Can you work these out from the model? Positions are in its coordinate system, mm. Face numbers are marked on the shaded views. Round coordinates to 2 decimals unless told otherwise and drop trailing zeros. Loops run counter-clockwise (first coordinate to the right, second up) from the corner with the lowest first, then second, coordinate; pieces in that order, holes last. Notation, with made-up numbers: M 45,81.5 L 49,81.5 A21 cw 49,87.5 Z; hole C -21.5,82 d10. An arc over 180 degrees is marked long. Use a Markdown table: item, result. Add a question column.
```python
from build123d import *

# Parameters (mm, degrees)
BOSS_EXTRUDE2_DEPTH = 160
SKETCH10_R          = 7.5
CUT_EXTRUDE3_DEPTH  = 37
SKETCH15_W          = 49.972994953
SKETCH15_H          = 20
BOSS_EXTRUDE3_DEPTH = 50
FILLET8_R           = 25
FILLET9_R           = 25
FILLET10_R          = 25
FILLET11_R          = 25
SKETCH20_R          = 12.5
CUT_EXTRUDE16_DEPTH = 120


with BuildPart() as part:
    # Sketch9 → Boss-Extrude2 (new body)
    with BuildSketch(Plane.XY):
        Polygon((-46.127266272, 8.011064826), (33.872733728, 7.400024977), (33.643600468, -22.599099976), (9.984036558, -22.418388271), (18.758604622, -7.484970869), (-31.242270425, -7.10306428), (-22.696835622, -22.168771831), (-46.356399532, -21.988060127), align=None)
    extrude(amount=-BOSS_EXTRUDE2_DEPTH)

    # Sketch10 → Cut-Extrude3 (cut)
    with BuildSketch(Plane(origin=(0.058494066, 7.658298076, 0), x_dir=(0.9999708317686696, -0.007637775322375965, 0), z_dir=(0.007637775322375965, 0.9999708317686696, 0))):
        with Locations(Location((-5.952514862, 19.602368066, 0), (0, 0, 180))):
            Circle(SKETCH10_R)
        with Locations(Location((-5.952514862, 140.397631934, 0), (0, 0, 180))):
            Circle(SKETCH10_R)
    extrude(amount=-CUT_EXTRUDE3_DEPTH, mode=Mode.SUBTRACT)

    # Sketch15 → Boss-Extrude3 (add)
    with BuildSketch(Plane(origin=(0.058494066, 7.658298076, 0), x_dir=(0.9999708317686696, -0.007637775322375965, 0), z_dir=(0.007637775322375965, 0.9999708317686696, 0))):
        with Locations((-6.171271485, 50)):
            Rectangle(SKETCH15_W, SKETCH15_H)
        with Locations((-6.171271485, 110)):
            Rectangle(SKETCH15_W, SKETCH15_H)
    extrude(amount=BOSS_EXTRUDE3_DEPTH)

    # Fillet8
    fillet8_edges = [part.edges().sort_by_distance(p)[0] for p in [
        (-30.716477311, 57.894815703, -50),
    ]]
    fillet(fillet8_edges, radius=FILLET8_R)

    # Fillet9
    # the kernel refuses this fillet: 25 mm, written as the material it takes off along each edge
    with BuildSketch(Plane(origin=(19.255060017, 57.513133196, -122.5), x_dir=(-0.9999708317686696, 0.007637775322376116, 0), z_dir=(0, 0, 1))) as fillet9_piece_1_section:
        with BuildLine():
            CenterArc((FILLET9_R, FILLET9_R), FILLET9_R, 180, 90)
            Line((0, FILLET9_R), (0, 0))
            Line((0, 0), (FILLET9_R, 0))
        make_face()
    fillet9_piece_1 = extrude(amount=145, mode=Mode.PRIVATE)
    fillet9_piece_1 = split(fillet9_piece_1, bisect_by=Plane(origin=(11.883432775, 50.243784792, -100), z_dir=(0, 0, 1)), keep=Keep.TOP, mode=Mode.PRIVATE)
    add(fillet9_piece_1, mode=Mode.SUBTRACT)

    # Fillet10
    fillet10_edges = [part.edges().sort_by_distance(p)[0] for p in [
        (-30.716477311, 57.894815703, -110),
    ]]
    fillet(fillet10_edges, radius=FILLET10_R)

    # Fillet11
    # the kernel refuses this fillet: 25 mm, written as the material it takes off along each edge
    with BuildSketch(Plane(origin=(19.255060017, 57.513133196, -37.5), x_dir=(-0.9999708317686696, 0.007637775322376116, 0), z_dir=(0, 0, -1))) as fillet11_piece_1:
        with BuildLine():
            CenterArc((FILLET11_R, -FILLET11_R), FILLET11_R, 90, 90)
            Line((0, -FILLET11_R), (0, 0))
            Line((0, 0), (FILLET11_R, 0))
        make_face()
    extrude(amount=145, mode=Mode.SUBTRACT)

    # Sketch20 → Cut-Extrude16 (cut)
    with BuildSketch(Plane(origin=(0, 0, -120), x_dir=(-1, 0, 0), z_dir=(0, 0, -1))):
        with Locations((5.9081509, 32.704600526)):
            Circle(SKETCH20_R)
    extrude(amount=-CUT_EXTRUDE16_DEPTH, mode=Mode.SUBTRACT)


solid = part.part
```
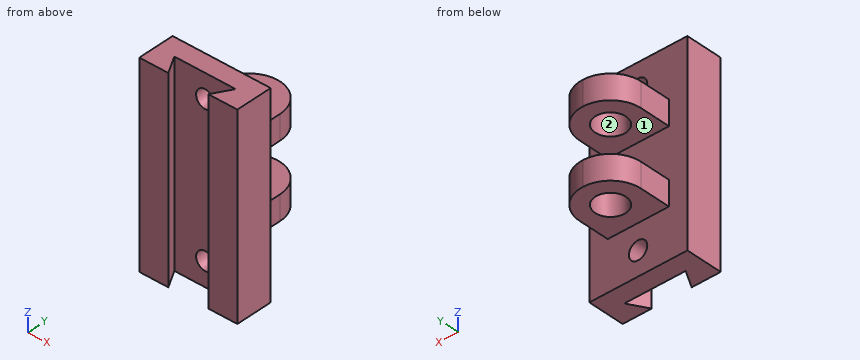
(1) If I drill on probe 1 along Z at (x, y) = (16, 19.5); probe 2 along Y at (x, z) = (16, -97); probe 3 along Y at (x, z) = (-24.5, -31) (3 decimals), over which ranges is the centre line in solid material (lowest first)? Write a range as [from, to].
(2) Suppose I cut it at A-A on z = -125. List the corners of the cut face in (x, y) for me.
(3) Suppose I cut it at C-C on x = -28. List the corners of the cut face in (y, z) for me.
(4) Suppose I cut it at B-B on y = 29. List the corners of the cut face in (x, z) for me.
(5) Suppose I cut it at D-D on z = -52.5. List the corners of the cut face in (x, y) for me, and give its area (3 significant figures).
(6) Thinking about a two-plate mould opening in Y: for the marked faces 1 and 2, which applies, released by +Y, released by -Y, zero draft, split by the parting line, or undercut?
(7) I'm going to push flat-ended pins straight in: pin 1 (3 mm diameter, centred on x = 9, y = 16, fed in from -Z); pin 2 (6 mm diameter, centred on y = 18.5, z = -52.5, fed in from -X); pin 3 (15 mm diameter, centred on x = -15, y = 38.5, fed in from +Z). Where does each tip first touch, or does it pass through?
Results below:
| question | item | result |
|---|---|---|
| 1 | probe 1 | z = [-120, -100], [-60, -40] |
| 1 | probe 2 | y = [-22.46, -12.18], [-7.46, 7.54] |
| 1 | probe 3 | y = [-22.155, -18.99], [-7.155, 7.846] |
| 2 | outline | M -46.36,-21.99 L -22.7,-22.17 L -31.24,-7.1 L 18.76,-7.48 L 9.98,-22.42 L 33.64,-22.6 L 33.87,7.4 L -46.13,8.01 Z |
| 3 | outline | M -22.13,-160 L -12.82,-160 L -12.82,0 L -22.13,0 Z; M -7.13,-160 L 7.87,-160 L 7.87,-120 L 44.41,-120 L 44.41,-100 L 7.87,-100 L 7.87,-60 L 44.41,-60 L 44.41,-40 L 7.87,-40 L 7.87,0 L -7.13,0 Z |
| 4 | outline | M -30.94,-120 L -17.85,-120 L -17.85,-100 L -30.94,-100 Z; M -30.94,-60 L -17.85,-60 L -17.85,-40 L -30.94,-40 Z; M 6.03,-120 L 19.04,-120 L 19.04,-100 L 6.03,-100 Z; M 6.03,-60 L 19.04,-60 L 19.04,-40 L 6.03,-40 Z |
| 5 | outline | M -46.36,-21.99 L -22.7,-22.17 L -31.24,-7.1 L 18.76,-7.48 L 9.98,-22.42 L 33.64,-22.6 L 33.87,7.4 L 18.87,7.51 L 19.06,32.51 A25 ccw -5.73,57.7 A25 ccw -30.91,32.9 L -31.1,7.9 L -46.13,8.01 Z; hole C -5.91,32.7 d25 |
| 5 | area | 3,520 mm² |
| 6 | face 1 | zero draft |
| 6 | face 2 | undercut |
| 7 | pin 1 | stops at z = -120 |
| 7 | pin 2 | stops at x = -31.04 |
| 7 | pin 3 | stops at z = -40 |
